```python
from build123d import *

# Parameters (mm, degrees)
F0_R     = 32.5
F1_DEPTH = 15
F2_R     = 5
F3_DEPTH = 14
F4_R     = 2


with BuildPart() as f1:
    # F0 (on Front) → F1 (new body)
    with BuildSketch(Plane.XZ):
        with BuildLine():
            ThreePointArc((10.9615384615, -46.217904264), (37.2620656763, -29.4582494649), (47.5, 0))
            ThreePointArc((47.5, 0), (37.2620656763, 29.4582494649), (10.9615384615, 46.217904264))
            ThreePointArc((10.9615384615, 46.217904264), (-47.5, 0), (10.9615384615, -46.217904264))
        make_face()
        Circle(F0_R, mode=Mode.SUBTRACT)
        with BuildLine():
            ThreePointArc((10.9615384615, 46.217904264), (37.2620656763, 29.4582494649), (47.5, 0))
            ThreePointArc((47.5, 0), (37.2620656763, -29.4582494649), (10.9615384615, -46.217904264))
            Line((10.9615384615, -46.217904264), (134.0384615385, -17.0276489394))
            ThreePointArc((134.0384615385, -17.0276489394), (112.5, 0), (134.0384615385, 17.0276489394))
            Line((134.0384615385, 17.0276489394), (10.9615384615, 46.217904264))
        make_face()
        with BuildLine():
            ThreePointArc((147.5, 0), (143.7281294597, 10.8530392766), (134.0384615385, 17.0276489394))
            ThreePointArc((134.0384615385, 17.0276489394), (112.5, 0), (134.0384615385, -17.0276489394))
            ThreePointArc((134.0384615385, -17.0276489394), (143.7281294597, -10.8530392766), (147.5, 0))
        make_face()
    extrude(amount=-F1_DEPTH)

    # F2 (on face) → F3 (join)
    with BuildSketch(Plane(origin=(10.9615384615, 0, 46.217904264), x_dir=(0.9730085108, 0, -0.2307692308), z_dir=(0.2307692308, 0, 0.9730085108))):
        with Locations((80.6287527084, 7.5)):
            Circle(F2_R)
    extrude(amount=F3_DEPTH)

    # F4
    f4_edges = [f1.edges().sort_by_distance(p)[0] for p in [
        (87.779728, 7.5, 42.387234),
    ]]
    fillet(f4_edges, radius=F4_R)


solid = f1.part
```
Model file for the job. Use its own axes, mm. Coordinates: 2 decimals unless noted, no trailing zeros. Loops run counter-clockwise (first coordinate to the right, second up) from the corner with the lowest first, then second, coordinate; pieces in that order, holes last. Notation, with made-up numbers: (-27.5, 29.5) - (-17.5, 29.5) arc R15 ccw to (-17.5, 49.5) - close; hole circle Ø11 at (67, 28.5). An arc over 180 degrees is marked (long way). Answer as a JSON object with one key per item and string values. Group by question number.
(1) Cut at A-A (x = -10.5). Give the cut face in (y, z), then the cut area to 3 significant figures.
(2) Two-plate mould, pull along Z, no slides. Class faces 1 (the face through (49, 15, 1)), 2 (the face through (71.638, 7.395, -31.827)), 3 (the face through (31, 7.4, 9.76)): released by +Z, released by -Z, zero draft, split by the parting line, or undercut.
(3) Cut at B-B (z = -30). Give the cut face in (x, y).
(4) Cut at C-C (z = -41). Give the cut face in (x, y).
(5) Flat gauge pins, fed straight in: pin 1 (1 mm diameter, centred on x = -12, y = 3.5, fed in from +Z); pin 2 (3 mm diameter, centred on y = 7, z = -8, fed in from -X); pin 3 (8 mm diameter, centred on x = 20, z = 23, fed in from -Y); pin 4 (2 mm diameter, centred on x = 101, y = 12, fed in from -Z). Where does each tip first touch, or does it go through?
(6) Probe line 1 along Z through (x, y) = (0, 12.25); line 2 along X through (y, z) = (12.5, 1); line 3 along Z through (x, y) = (-17.5, 13). List the from-to ranges inside material, lowest first.
Geometry says:
{
 "1": {"outline": "(0, -46.32) - (15, -46.32) - (15, -30.76) - (0, -30.76) - close; (0, 30.76) - (15, 30.76) - (15, 46.32) - (0, 46.32) - close", "area": "467 mm^2"},
 "2": {"face 1": "zero draft", "face 2": "released by -Z", "face 3": "undercut"},
 "3": {"outline": "(-36.83, 0) - (-12.5, 0) - (-12.5, 15) - (-36.83, 15) - close; (12.5, 0) - (79.34, 0) - (79.34, 15) - (12.5, 15) - close"},
 "4": {"outline": "(-23.98, 0) - (32.96, 0) - (32.96, 15) - (-23.98, 15) - close"},
 "5": {"pin 1": "stops at z = 46.09", "pin 2": "stops at x = -47.05", "pin 3": "stops at y = 0", "pin 4": "stops at z = -25.1"},
 "6": {"line 1": "z = -47.5 to -32.5, 32.5 to 47.5", "line 2": "x = -47.49 to -32.48, 32.48 to 147.47", "line 3": "z = -44.16 to -27.39, 27.39 to 44.16"}
}
